```python
from build123d import *

# Parameters (mm, degrees)
SALIENTE_EXTRUIR3_DEPTH = 6.35
CROQUIS5_W              = 2.54
CROQUIS5_H              = 196.85
CORTAR_EXTRUIR1_DEPTH   = 6.35
CROQUIS6_W              = 6.35
CROQUIS6_H              = 196.85
CROQUIS6_W_2            = 76.2
CROQUIS6_H_2            = 6.35
CORTAR_EXTRUIR2_DEPTH   = 7.35
CROQUIS7_W              = 3.81
CROQUIS7_H              = 196.85
SALIENTE_EXTRUIR5_DEPTH = 6.35
CROQUIS8_W              = 76.2
CROQUIS8_H              = 3.81
SALIENTE_EXTRUIR6_DEPTH = 6.35


with BuildPart() as part:
    # Croquis2 → Saliente-Extruir3 (new body)
    with BuildSketch(Plane.XY):
        with BuildLine():
            Line((0, 0), (6.35, 0))
            Line((6.35, 0), (6.35, -6.35))
            Line((6.35, -6.35), (82.55, -6.35))
            Line((82.55, -6.35), (82.55, 0))
            Line((82.55, 0), (88.9, 0))
            Line((88.9, 0), (88.9, 50.8))
            ThreePointArc((88.9, 50.8), (83.320384182, 64.270384182), (69.85, 69.85))
            Line((69.85, 69.85), (63.5, 69.85))
            ThreePointArc((63.5, 69.85), (50.029615818, 75.429615818), (44.45, 88.9))
            Line((44.45, 88.9), (44.45, 190.5))
            ThreePointArc((44.45, 190.5), (38.870384182, 203.970384182), (25.4, 209.55))
            Line((25.4, 209.55), (0, 209.55))
            Line((0, 209.55), (0, 203.2))
            Line((0, 203.2), (-6.35, 203.2))
            Line((-6.35, 203.2), (-6.35, 6.35))
            Line((-6.35, 6.35), (0, 6.35))
            Line((0, 6.35), (0, 0))
        make_face()
    extrude(amount=SALIENTE_EXTRUIR3_DEPTH)

    # Croquis5 → Cortar-Extruir1 (cut)
    with BuildSketch(Plane.ZY.offset(6.35)):
        with Locations((1.27, 104.775)):
            Rectangle(CROQUIS5_W, CROQUIS5_H)
    extrude(amount=-CORTAR_EXTRUIR1_DEPTH, mode=Mode.SUBTRACT)


with BuildPart() as part_1:
    # Sólido-Mover/Copiar1: moved
    add(part.part.moved(Location((-148.301048564, -44.960118156, 222.608991853))))

    # Croquis6 → Cortar-Extruir2 (cut, through all)
    with BuildSketch(Plane.XY.offset(228.958991853)):
        with Locations((-151.476048564, 59.814881844)):
            Rectangle(CROQUIS6_W, CROQUIS6_H)
        with Locations((-103.851048564, -48.135118156)):
            Rectangle(CROQUIS6_W_2, CROQUIS6_H_2)
    extrude(amount=-CORTAR_EXTRUIR2_DEPTH, mode=Mode.SUBTRACT)

    # Croquis7 → Saliente-Extruir5 (add)
    with BuildSketch(Plane.ZY.offset(148.301048564)):
        with Locations((224.513991853, 59.814881844)):
            Rectangle(CROQUIS7_W, CROQUIS7_H)
    extrude(amount=SALIENTE_EXTRUIR5_DEPTH)

    # Croquis8 → Saliente-Extruir6 (add)
    with BuildSketch(Plane(origin=(0, -44.960118156, 0), x_dir=(-1, 0, 0), z_dir=(0, -1, 0))):
        with Locations((103.851048564, -224.513991853)):
            Rectangle(CROQUIS8_W, CROQUIS8_H)
    extrude(amount=SALIENTE_EXTRUIR6_DEPTH)


solid = part_1.part
```
The listing builds one solid part. Answer for the finished solid, in the listing's coordinates (mm). A direction names the side the tool comes from. Give positions to 0.01 mm unless a question says otherwise; leave off trailing zeros. Order: outer loops, then holes, each group sorted by start corner. A loop starts at its lowest first (then second) coordinate and runs counter-clockwise, first axis right, second up.
1) Find section C-C on y = 110. Write down the section's boundary in (x, z), then the cut area to 3 significant figures.
Reported:
outline: (-154.65, 222.61) - (-103.85, 222.61) - (-103.85, 228.96) - (-148.3, 228.96) - (-148.3, 226.42) - (-154.65, 226.42) - close
area: 306 mm2
2) Consider line 1 along X through (y, z) = (85, 226.25); line 2 along X through (y, z) = (106, 228); line 3 along Y through (x, z) = (-124, 227.5). Determine where each line is inside the solid, lowest interval first.
Reported:
line 1: x = -154.65 to -103.85
line 2: x = -148.3 to -103.85
line 3: y = -44.96 to 164.59
3) Find section A-A on z = 227.5. Write down the section's boundary in (x, y).
Reported:
outline: (-148.3, -44.96) - (-59.4, -44.96) - (-59.4, 5.84) arc R19.05 ccw to (-78.45, 24.89) - (-84.8, 24.89) arc R19.05 cw to (-103.85, 43.94) - (-103.85, 145.54) arc R19.05 ccw to (-122.9, 164.59) - (-148.3, 164.59) - close
4) Given P1, Ø3, axis at y = 127.5, z = 225, coming from the +X side; P2, Ø1.9, axis at x = -104, y = -49.5, coming from the +Z side; P3, Ø1.9, axis at y = -48, z = 223.5, coming from the +X side, each flat-ended and moving along its own axis, determine where each tip first touches the part or whether it passes through.
Reported:
P1: stops at x = -103.85
P2: stops at z = 226.42
P3: stops at x = -65.75
5) For faces 1 (the face through (-151, 58, 226.419)), 2 (the face through (-151, 158.24, 224)), 3 (the face through (-65.751, -48, 225)), 4 (the face through (-103.851, 94, 226)), determine the directions among +Z, -Z, +X, -X, +Y, -Y from which every point of the face is accessible in a straight line to the end or side of a thin tool.
Reported:
face 1: +Z, -X, +Y, -Y
face 2: +Z, -Z, -X, +Y
face 3: +Z, -Z, +X, -Y
face 4: +Z, -Z, +X, +Y
6) Find section B-B on y = -27. Write down the section's boundary in (x, z).
Reported:
outline: (-154.65, 222.61) - (-59.4, 222.61) - (-59.4, 228.96) - (-148.3, 228.96) - (-148.3, 226.42) - (-154.65, 226.42) - close
